Part model, mm, in its own coordinate system. Round coordinates to 2 decimals unless told otherwise and drop trailing zeros. Write each loop counter-clockwise with the first axis right and the second up, starting at its lowest first coordinate (ties: lowest second). Pieces come first, ordered by that corner, then holes. Notation, with made-up numbers: (82.5, 71.5) -> (105.5, 71.5) arc R14 ccw to (105.5, 97.5) -> close; hole circle Ø2 at (61.25, 2.25). An arc over 180 degrees is marked (long way). Use CSV: the item, a comma, the result in double quotes. Start each with the question number.
(1) Saw through at C-C (x = -71.12). Give the cut face in (y, z).
(2) Saw through at D-D (y = -25). Give the cut face in (x, z), plus the area to 3 significant figures.
(3) Saw through at A-A (y = 23.5). Give the cut face in (x, z).
(4) Probe line 1 (X direction, y = 29, z = -73.5); line 2 (Y direction, x = -48.5, z = -40.5); line 3 (X direction, y = 20, z = -83.5). List the from-to ranges inside material, lowest first. Write a range as [from, to].
(5) Two-plate mould, pull along X, no slides. Class faces 1 (the flat face through (-1, -31.75, -50)), 2 (the cylindrical face through (-98.09, 0.92, -50.09)), 3 (the flat face through (50.8, 0, -50)): released by +X, released by -X, zero draft, split by the parting line, or undercut.
(6) Drop flat-ended pins along their axis: pin 1 (8 mm diameter, centred on x = -50, y = -8, fed in from +Z); pin 2 (5.5 mm diameter, centred on y = 24, z = -66.5, fed in from -X); pin 3 (4 mm diameter, centred on x = -82, z = -20.5, fed in from +Y); pin 4 (1 mm diameter, centred on y = -4.5, z = -84, fed in from -X). Give the stop position or say it passes through.
```python
from build123d import *

# Parameters (mm, degrees)
F1_DEPTH = 101.6


with BuildPart() as f1:
    # F0 (on Top) → F1 (new body)
    with BuildSketch(Plane.XY):
        with BuildLine():
            ThreePointArc((50.8, 29.21), (50.0560512242, 31.0060512242), (48.26, 31.75))
            Line((48.26, 31.75), (-48.26, 31.75))
            ThreePointArc((-48.26, 31.75), (-50.0560512242, 31.0060512242), (-50.8, 29.21))
            Line((-50.8, 29.21), (-50.8, 17.7601451641))
            ThreePointArc((-50.8, 17.7601451641), (-45.8543003634, 9.4852294714), (-44.1325, 0))
            ThreePointArc((-44.1325, 0), (-45.8543003634, -9.4852294714), (-50.8, -17.7601451641))
            Line((-50.8, -17.7601451641), (-50.8, -29.21))
            ThreePointArc((-50.8, -29.21), (-50.0560512242, -31.0060512242), (-48.26, -31.75))
            Line((-48.26, -31.75), (48.26, -31.75))
            ThreePointArc((48.26, -31.75), (50.0560512242, -31.0060512242), (50.8, -29.21))
            Line((50.8, -29.21), (50.8, 29.21))
        make_face()
        with BuildLine():
            ThreePointArc((-44.1325, 0), (-45.8543003634, 9.4852294714), (-50.8, 17.7601451641))
            Line((-50.8, 17.7601451641), (-50.8, -17.7601451641))
            ThreePointArc((-50.8, -17.7601451641), (-45.8543003634, -9.4852294714), (-44.1325, 0))
        make_face()
        with BuildLine():
            Line((-50.8, -17.7601451641), (-50.8, 17.7601451641))
            ThreePointArc((-50.8, 17.7601451641), (-98.1075, 0), (-50.8, -17.7601451641))
        make_face()
    extrude(amount=-F1_DEPTH)


solid = f1.part
```
Answers:
1,outline,"(-26.99, -101.6) -> (26.99, -101.6) -> (26.99, 0) -> (-26.99, 0) -> close"
2,outline,"(-81.28, -101.6) -> (-60.96, -101.6) -> (-60.96, 0) -> (-81.28, 0) -> close; (-50.8, -101.6) -> (50.8, -101.6) -> (50.8, 0) -> (-50.8, 0) -> close"
2,area,"12,400 mm²"
3,outline,"(-84.39, -101.6) -> (-57.85, -101.6) -> (-57.85, 0) -> (-84.39, 0) -> close; (-50.8, -101.6) -> (50.8, -101.6) -> (50.8, 0) -> (-50.8, 0) -> close"
4,line 1,"x = [-50.8, 50.8]"
4,line 2,"y = [-31.74, 31.74]"
4,line 3,"x = [-89.24, -53], [-50.8, 50.8]"
5,face 1,"zero draft"
5,face 2,"undercut"
5,face 3,"released by +X"
6,pin 1,"stops at z = 0"
6,pin 2,"stops at x = -87.76"
6,pin 3,"stops at y = 25.48"
6,pin 4,"stops at x = -97.81"
